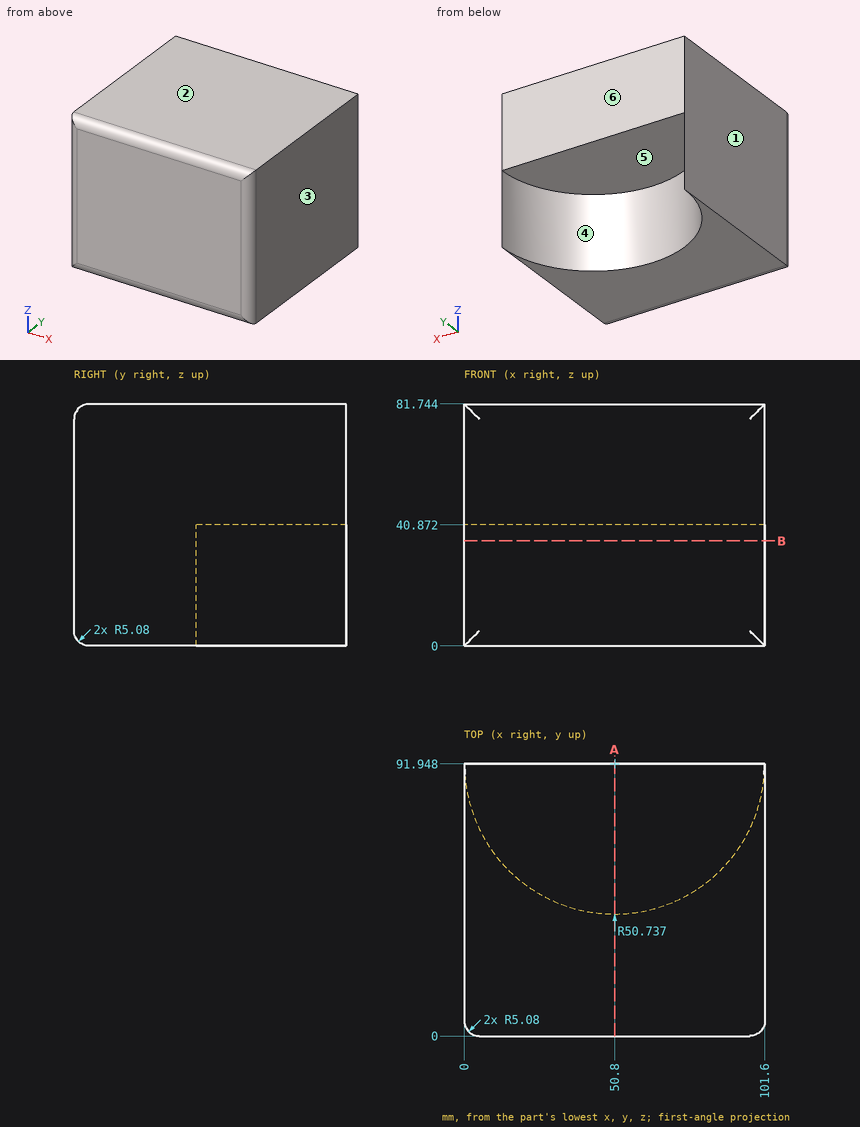
Answer from the drawing. Dimensions are ordinates in mm from the lowest x, y and z of the part. A direction names the side the tool comes from. Coordinates: 2 decimals unless noted, no trailing zeros. Write each loop counter-clockwise with the first axis right and the second up, starting at its lowest first coordinate (ties: lowest second). Pieces come first, ordered by that corner, then holes. Notation, with made-up numbers: M 85,33.25 L 124,33.25 A27 cw 124,67.25 Z; hole C 31,62 d3. An arc over 180 degrees is marked long. Put each result on its own line as item: value. Start each with the question number.
1. A flat-ended cylindrical pin translates along its axis: P1, Ø15, axis at x = 65.5, y = 54, coming from the -Z side. Find the tip coordinate at first contact, or state that the pin passes through.
2. A cutting plane is placed at A-A on x = 50.8. Write down the section's boundary in (y, z), then the cut area to 3 significant figures.
3. Which of the six approach directions +Z, -Z, +X, -X, +Y, -Y give full straight-line access (tool end or side, diameter ignored) to the marked faces 5 and 6?
4. Consider line 1 (Z direction, x = 28, y = 88); line 2 (X direction, y = 73, z = 10); line 3 (Y direction, x = 56.5, z = 34.5). Determine where each line is inside the solid, lowest interval first. Write a range as from..to.
5. For a pull along X with two mould halves and no side action, classify the marked faces 1, 2, 3 and 4 as pulls with the +X half, pulls with the -X half, needs draft (parallel to the pull), parting line crosses it, or undercut.
6. A cutting plane is placed at B-B on z = 35.5. Write down the section's boundary in (x, y).
Resolved:
1. P1: stops at z = 40.87
2. outline: M 0,5.08 A5.08 ccw 5.08,0 L 41.21,0 L 41.21,40.87 L 91.95,40.87 L 91.95,81.74 L 5.08,81.74 A5.08 ccw 0,76.66 Z
2. area: 5,430 mm2
3. face 5: -Z, +Y
3. face 6: +Z, -Z, +X, -X, +Y
4. line 1: z = 40.87..81.74
4. line 2: x = 0..3.73, 97.87..101.6
4. line 3: y = 0..41.53
5. face 1: pulls with the -X half
5. face 2: needs draft
5. face 3: pulls with the +X half
5. face 4: undercut
6. outline: M 0,5.08 A5.08 ccw 5.08,0 L 96.52,0 A5.08 ccw 101.6,5.08 L 101.6,91.95 L 101.54,91.95 A50.74 cw 0.06,91.95 L 0,91.95 Z
